Check sheet for the modelled part. Datum: model origin and axes. Units: mm. Face numbers are marked on the shaded views. A direction names the side the tool comes from. Round coordinates to 2 decimals unless told otherwise and drop trailing zeros. Order: outer loops, then holes, each group sorted by start corner. A loop starts at its lowest first (then second) coordinate and runs counter-clockwise, first axis right, second up. Notation, with made-up numbers: (45, 41) -> (86, 41) arc R23 ccw to (86, 75) -> close; hole circle Ø5 at (-36, 84). An arc over 180 degrees is marked (long way). Answer in a Markdown table with one row per item.
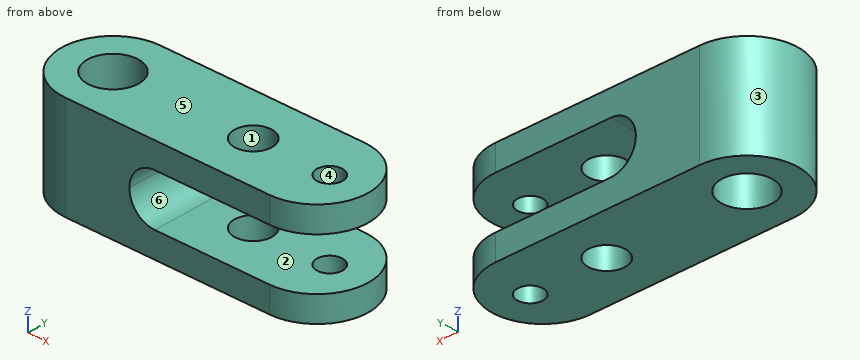
```python
from build123d import *

# Parameters (mm, degrees)
BOSS_EXTRUDE1_DEPTH = 12.7
SKETCH2_R           = 3.175
SKETCH2_R_2         = 4.6355
SKETCH2_R_3         = 6.35
CUT_EXTRUDE1_DEPTH  = 25.4
SKETCH3_W           = 47.625
SKETCH3_H           = 12.7
CUT_EXTRUDE2_DEPTH  = 25.4
FILLET1_R           = 6.35


with BuildPart() as part:
    # Sketch1 → Boss-Extrude1 (new, symmetric)
    with BuildSketch(Plane.XY):
        with BuildLine():
            Line((-25.4, 12.7), (25.4, 12.7))
            ThreePointArc((25.4, 12.7), (38.1, 0), (25.4, -12.7))
            Line((25.4, -12.7), (-25.4, -12.7))
            ThreePointArc((-25.4, -12.7), (-38.1, 0), (-25.4, 12.7))
        make_face()
    extrude(amount=BOSS_EXTRUDE1_DEPTH, both=True)

    # Sketch2 → Cut-Extrude1 (cut)
    with BuildSketch(Plane.XY.offset(12.7)):
        with Locations((28.575, 0)):
            Circle(SKETCH2_R)
        with Locations((9.525, 0)):
            Circle(SKETCH2_R_2)
        with Locations((-25.4, 0)):
            Circle(SKETCH2_R_3)
    extrude(amount=-CUT_EXTRUDE1_DEPTH, mode=Mode.SUBTRACT)

    # Sketch3 → Cut-Extrude2 (cut)
    with BuildSketch(Plane(origin=(0, 12.7, 0), x_dir=(1, 0, 0), z_dir=(0, 1, 0))):
        with Locations((14.2875, 0)):
            Rectangle(SKETCH3_W, SKETCH3_H)
    extrude(amount=-CUT_EXTRUDE2_DEPTH, mode=Mode.SUBTRACT)

    # Fillet1
    fillet1_edges = [part.edges().sort_by_distance(p)[0] for p in [
        (-9.525, 0, -6.35),
        (-9.525, 0, 6.35),
    ]]
    fillet(fillet1_edges, radius=FILLET1_R - 0.0001)  # a hair under: the kernel refuses the full size


solid = part.part
```
(1) Section check A-A on y = 0. Give the number of separate pieces and of enclosed holes in the cut face, plus the area to 3 significant figures.
Solutions:
| item | result |
|---|---|
| separate pieces | 6 |
| enclosed holes | 0 |
| area | 827 mm^2 |
(2) Section check C-C on x = 0.5. Record the boundary of the cut face in (y, z).
Solutions:
| item | result |
|---|---|
| outline | (-12.7, -12.7) -> (12.7, -12.7) -> (12.7, -6.35) -> (-12.7, -6.35) -> close; (-12.7, 6.35) -> (12.7, 6.35) -> (12.7, 12.7) -> (-12.7, 12.7) -> close |
(3) Depth check by flat-ended pin: pin 1 Ø14.5 at (x, y) = (-25.4, 0) entering from -Z; pin 2 Ø3 at (x, z) = (28, 9) entering from -Y; pin 3 Ø2 at (y, z) = (-3.5, -8.5) entering from -X. Enter the tip coordinate at first touch or a pass-through.
Solutions:
| item | result |
|---|---|
| pin 1 | z = -12.7 |
| pin 2 | y = -12.65 |
| pin 3 | x = -37.85 |
(4) Tool access check on the marked faces 5 and 6. Record the directions out of +Z, -Z, +X, -X, +Y, -Y that give a thin tool (end or side, any length) a straight path to the whole face; none if there is none.
Solutions:
| item | result |
|---|---|
| face 5 | +Z, +X, -X, +Y, -Y |
| face 6 | +X, +Y, -Y |
(5) Draft check along Y on the marked faces 1, 2, 3 and 4. Enter one of: pulls with the +Y half, pulls with the -Y half, needs draft (parallel to the pull), parting line crosses it, or undercut.
Solutions:
| item | result |
|---|---|
| face 1 | undercut |
| face 2 | needs draft |
| face 3 | parting line crosses it |
| face 4 | undercut |
(6) Section check D-D on z = -4.25. Record the boundary of the cut face in (x, y).
Solutions:
| item | result |
|---|---|
| outline | (-25.4, -12.7) -> (-7.89, -12.7) -> (-7.89, 12.7) -> (-25.4, 12.7) arc R12.7 ccw to start; hole circle Ø12.7 at (-25.4, 0) |
(7) Scan lines: probe 1 along X at (y, z) = (0.25, 7.5); probe 2 along X at (y, z) = (0.25, 0.25); probe 3 along Y at (x, z) = (-25.4, -0.75). Record each from-to range of solid material in increasing order. Write a range as from..to.
Solutions:
| item | result |
|---|---|
| probe 1 | -38.1..-31.75, -19.05..4.9, 14.15..25.41, 31.74..38.1 |
| probe 2 | -38.1..-31.75, -19.05..-9.52 |
| probe 3 | -12.7..-6.35, 6.35..12.7 |
